from build123d import *

# Parameters (mm, degrees)
SKETCH1_R           = 40
SKETCH1_R_2         = 1.5
SKETCH1_R_3         = 5
BOSS_EXTRUDE1_DEPTH = 5
FILLET2_R           = 10


with BuildPart() as part:
    # Sketch1 → Boss-Extrude1 (new body)
    with BuildSketch(Plane(origin=(0, 0, 0), x_dir=(1, 0, 0), z_dir=(0, 1, 0))):
        with Locations(Location((0, 0, 0), (0, 0, 270))):
            Circle(SKETCH1_R)
        with Locations(Location((-15.5, 15.5, 0), (0, 0, 270))):
            Circle(SKETCH1_R_2, mode=Mode.SUBTRACT)
        with Locations(Location((15.5, 15.5, 0), (0, 0, 270))):
            Circle(SKETCH1_R_2, mode=Mode.SUBTRACT)
        with Locations(Location((-15.5, -15.5, 0), (0, 0, 270))):
            Circle(SKETCH1_R_2, mode=Mode.SUBTRACT)
        with Locations(Location((15.5, -15.5, 0), (0, 0, 270))):
            Circle(SKETCH1_R_2, mode=Mode.SUBTRACT)
        with Locations(Location((0, 0, 0), (0, 0, 270))):
            Circle(SKETCH1_R_3, mode=Mode.SUBTRACT)
    extrude(amount=BOSS_EXTRUDE1_DEPTH)

    # Fillet2
    # the kernel refuses this fillet: 10 mm, written as the material it takes off along each edge
    with BuildSketch(Plane(origin=(0, 5, 0), x_dir=(0, 0, 1), z_dir=(-1, 0, 0))) as fillet2_piece_1:
        with BuildLine():
            CenterArc((31.339745962, -10), FILLET2_R, 30, 60)
            Line((31.339745962, 0), (31.339745962, 0.2))
            Line((31.339745962, 0.2), (40, 0.2))
            Line((40, 0.2), (40.2, 0))
            ThreePointArc((40.2, 0), (40.2, -2.5), (40.173205081, -4.9))
            Line((40.173205081, -4.9), (40, -5))
        make_face()
    revolve(axis=Axis((0, 5, 0), (0, 1, 0)), mode=Mode.SUBTRACT)


solid = part.part
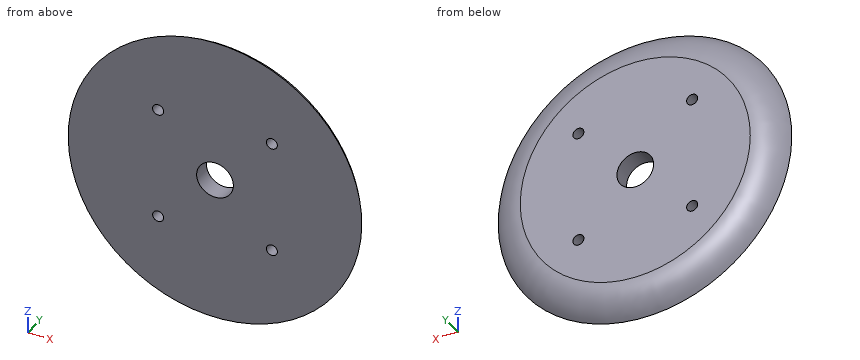
The listing builds one solid part. Answer for the finished solid, in the listing's coordinates (mm). Give positions to 0.01 mm unless a question says otherwise; leave off trailing zeros. Order: outer loops, then holes, each group sorted by start corner. A loop starts at its lowest first (then second) coordinate and runs counter-clockwise, first axis right, second up. Notation, with made-up numbers: (84, -31) -> (108, -31) arc R29 cw to (108, 0) -> close; hole circle Ø10 at (69.25, 8.5). An arc over 180 degrees is marked (long way). Put each result on its own line as item: value.
Item 1: A cutting plane is placed at C-C on x = 15.5. Count the separate pieces of the cut face and the enclosed holes in it, plus the area to 3 significant figures.
Established:
separate pieces: 3
enclosed holes: 0
area: 311 mm^2
Item 2: A cutting plane is placed at A-A on z = 0. Give the vertices of the cut face in (x, y), plus the area to 3 significant figures.
Established:
outline: (-40, 0) -> (-5, 0) -> (-5, 5) -> (-31.34, 5) arc R10 ccw to start; (5, 0) -> (40, 0) arc R10 ccw to (31.34, 5) -> (5, 5) -> close
area: 325 mm^2
Item 3: Given P1, Ø1, axis at x = -17.5, y = 4.5, coming from the -Z side; P2, Ø8, axis at x = 12.5, z = 30.5, coming from the -Y side; P3, Ø2.5, axis at x = -15.5, z = -15.5, coming from the +Y side; P4, Ø1, axis at y = 2, z = 30.5, coming from the +X side, each flat-ended and moving along its own axis, determine where each tip first touches the part or whether it passes through.
Established:
P1: stops at z = -31.15
P2: stops at y = 0
P3: passes through
P4: stops at x = 24.45
Item 4: A cutting plane is placed at B-B on y = 2.2. Give the vertices of the cut face in (x, z), plus the area to 3 significant figures.
Established:
outline: circle Ø76.56 at (0, 0); hole circle Ø3 at (-15.5, -15.5); hole circle Ø3 at (-15.5, 15.5); hole circle Ø10 at (0, 0); hole circle Ø3 at (15.5, -15.5); hole circle Ø3 at (15.5, 15.5)
area: 4,500 mm^2
Item 5: Straight lines are drawn through the part: line 1 (X direction, y = 2.2, z = -16.5); line 2 (X direction, y = 3.75, z = -15.5); line 3 (X direction, y = 2.7, z = 0). For each, find the intervals that lie inside material, in ascending order.
Established:
line 1: x = -34.54 to -16.62, -14.38 to 14.38, 16.62 to 34.54
line 2: x = -32.69 to -17, -14 to 14, 17 to 32.69
line 3: x = -37.72 to -5, 5 to 37.72
